Geometry check sheet. Reference: the model listing, model coordinates, mm. A direction names the side the tool comes from. Round coordinates to 2 decimals unless told otherwise and drop trailing zeros. Loops run counter-clockwise (first coordinate to the right, second up) from the corner with the lowest first, then second, coordinate; pieces in that order, holes last. Notation, with made-up numbers: (22, -21) -> (48, -21) arc R27 cw to (48, -2) -> close; hole circle Ø8 at (86.5, 14.5). An arc over 180 degrees is marked (long way). Use a Markdown table: item, result. Add a question column.
Q1. Gauge pin test, flat ends, axial feed: P1, Ø3, axis at x = 16, z = 5, coming from the +Y side; P2, Ø3, axis at x = 2.5, z = 2.5, coming from the -Y side; P3, Ø3.5, axis at x = 9.5, z = 3.9, coming from the -Y side; P4, Ø1.5, axis at y = -1.5, z = 5.5, coming from the +X side. Record the tip position at first contact, or that the pin passes through.
Q2. Sectioned sample at A-A, the plane z = 3.9. Enter the section's corners in (x, y), then the cut area to 4 significant figures.
Q3. Set-up check for faces 4 (the face through (16, 0, 4)), 5 (the face through (3, 0, 4)), 6 (the face through (9, 2, 7.8)): record each of +Z, -Z, +X, -X, +Y, -Y from which the full face is reachable in a straight line by a thin tool's end or side.
Q4. Sectioned sample at D-D, the plane z = 7.5. Enter the section's corners in (x, y).
Q5. Sectioned sample at C-C, the plane y = 3.5. Enter the section's corners in (x, z), then the cut area to 3 significant figures.
Q6. Material ranges on L1, parallel to X at y = 2.25, z = 3.9; L2, parallel to X at y = -0.25, z = 3.9; L3, parallel to Y at x = 3.75, z = 1.5, recorded low to high.
Q7. Release check for a two-part mould opening along X. For faces 1 (the face through (17.274, 4.232, 3.845)), 2 (the face through (9.6, 1.2, 6.9)), 3 (the face through (1.774, 4.268, 3.845)) record: released by +X, released by -X, zero draft, split by the parting line, or undercut.
Q8. Sectioned sample at B-B, the plane x = 9.5. Enter the section's corners in (y, z), then the cut area to 3 significant figures.
```python
from build123d import *

# Parameters (mm, degrees)
EXTRUDE_2_DEPTH     = 7.8
SKETCH_3_W          = 7.8
SKETCH_3_H          = 7.8
EXTRUDE_3_DEPTH     = 3
CUT_EXTRUDE_1_REACH = 24.228
SKETCH_4_R          = 3


with BuildPart() as part:
    # 草图2 → 凸台-拉伸2 (new body)
    with BuildSketch(Plane.XY):
        Polygon((0, 0), (19, 0), (19, 3), (15.5, 5.5), (3.5, 5.5), (0, 3), align=None)
    extrude(amount=EXTRUDE_2_DEPTH)

    # 草图3 → 凸台-拉伸3 (add)
    with BuildSketch(Plane(origin=(0, 0, 0), x_dir=(-1, 0, 0), z_dir=(0, -1, 0))):
        with Locations((-9.5, -3.9)):
            Rectangle(SKETCH_3_W, SKETCH_3_H)
    extrude(amount=EXTRUDE_3_DEPTH)

    # 草图4 → 切除-拉伸1 (cut, up to next)
    with BuildSketch(Plane(origin=(0, -3, 0), x_dir=(-1, 0, 0), z_dir=(0, -1, 0)), mode=Mode.PRIVATE) as cut_extrude_1_sk1:
        with Locations(Location((-9.5, -3.9, 0), (0, 0, 90))):
            Circle(SKETCH_4_R)
    cut_extrude_1_tool1 = extrude(cut_extrude_1_sk1.sketch, amount=-CUT_EXTRUDE_1_REACH, mode=Mode.PRIVATE) & part.part
    add(cut_extrude_1_tool1.solids().sort_by_distance((9.5, -3, 3.9))[0], mode=Mode.SUBTRACT)


solid = part.part
```
Values:
| question | item | result |
|---|---|---|
| 1 | P1 | y = 5.5 |
| 1 | P2 | y = 0 |
| 1 | P3 | through |
| 1 | P4 | x = 13.4 |
| 2 | outline | (0, 0) -> (5.6, 0) -> (5.6, -3) -> (6.5, -3) -> (6.5, 5.5) -> (3.5, 5.5) -> (0, 3) -> close; (12.5, -3) -> (13.4, -3) -> (13.4, 0) -> (19, 0) -> (19, 3) -> (15.5, 5.5) -> (12.5, 5.5) -> close |
| 2 | area | 68.15 mm^2 |
| 3 | face 4 | +Z, -Z, +X, -Y |
| 3 | face 5 | +Z, -Z, -X, -Y |
| 3 | face 6 | +Z, +X, -X, +Y, -Y |
| 4 | outline | (0, 0) -> (5.6, 0) -> (5.6, -3) -> (13.4, -3) -> (13.4, 0) -> (19, 0) -> (19, 3) -> (15.5, 5.5) -> (3.5, 5.5) -> (0, 3) -> close |
| 5 | outline | (0.7, 0) -> (18.3, 0) -> (18.3, 7.8) -> (0.7, 7.8) -> close; hole circle Ø6 at (9.5, 3.9) |
| 5 | area | 109 mm^2 |
| 6 | L1 | 0 to 6.5, 12.5 to 19 |
| 6 | L2 | 5.6 to 6.5, 12.5 to 13.4 |
| 6 | L3 | 0 to 5.5 |
| 7 | face 1 | released by +X |
| 7 | face 2 | undercut |
| 7 | face 3 | released by -X |
| 8 | outline | (-3, 0) -> (5.5, 0) -> (5.5, 0.9) -> (-3, 0.9) -> close; (-3, 6.9) -> (5.5, 6.9) -> (5.5, 7.8) -> (-3, 7.8) -> close |
| 8 | area | 15.3 mm^2 |
